Read the model definition and answer for the solid it produces. Units are mm, in the model's axes. A direction names the side the tool comes from. Coordinates: 2 decimals unless noted, no trailing zeros. Write each loop counter-clockwise with the first axis right and the second up, starting at its lowest first coordinate (ties: lowest second). Pieces come first, ordered by that corner, then holes.
(1) Section D-D on z = 4.75 is taken. State how many separate pieces and enclosed holes the cut face has, then the cut area to 3 significant figures.
(2) Given pin 1 (1 mm diameter, centred on y = -11, z = 1, fed in from +X); pin 2 (1.5 mm diameter, centred on x = 27, z = 0.5, fed in from -Y); pin 3 (1.8 mm diameter, centred on x = 4.5, z = 4, fed in from +Y), each flat-ended and moving along its own axis, determine where each tip first touches the part or whether it passes through.
(3) Find the intervals of material crossed by probe 1 along X at (y, z) = (-18, 4.25); probe 2 along X at (y, z) = (-8, 2.75); probe 3 along Y at (x, z) = (9, 1), in increasing order.
(4) Section A-A on y = 3 is taken. Write down the section's boundary in (x, z).
(5) The mould has two halves that part along X. Classify faces 4 (the flat face through (63.013, 1.422, 2.958)), 5 (the flat face through (3, -11, 0)), 6 (the cylindrical face through (-29.21, -4.43, 3.04)): +X half, -X half, draft (parallel to the pull), parting line (faces both ways), or undercut.
(6) Section C-C on x = 23 is taken. Write down the section's boundary in (y, z).
(7) Section B-B on x = -35.5 is taken. Write down the section's boundary in (y, z).
(8) Which of the six approach directions +Z, -Z, +X, -X, +Y, -Y give full straight-line access (tool end or side, diameter ignored) to faces 1 (the flat face through (56.063, -8.065, 3.042)), 2 (the cylindrical face through (-36.754, 13.724, 2.958)), 3 (the flat face through (-47.563, -31.236, 2.958))?
from build123d import *

# Parameters (mm, degrees)
SKETCH1_R                = 4.05
BOSS_EXTRUDE1_DEPTH      = 6
M4_CLEARANCE_HOLE1_D     = 4.5
M4_CLEARANCE_HOLE1_DEPTH = 80.96
M4_CLEARANCE_HOLE1_TIP   = 1.351936393
CUT_EXTRUDE1_DEPTH       = 103.314309644


with BuildPart() as part:
    # Sketch1 → Boss-Extrude1 (new body)
    with BuildSketch(Plane.XY):
        with BuildLine():
            Line((-65.19060966, -38.213571923), (-29.435009511, -24.059676563))
            ThreePointArc((-29.435009511, -24.059676563), (-26.147647316, -23.075006142), (-22.740346385, -22.666807174))
            Line((-22.740346385, -22.666807174), (18.034765948, -21.307032913))
            ThreePointArc((18.034765948, -21.307032913), (21.515927007, -21.494956503), (24.911568818, -22.284522385))
            Line((24.911568818, -22.284522385), (74.630790843, -38.525664943))
            ThreePointArc((74.630790843, -38.525664943), (93.086798158, -30.149764409), (86.35131748, -11.033979941))
            Line((86.35131748, -11.033979941), (39.011755224, 14.232375332))
            ThreePointArc((39.011755224, 14.232375332), (34.124223209, 16.06850435), (28.928004649, 16.57708242))
            Line((28.928004649, 16.57708242), (-31.672918815, 14.556154182))
            ThreePointArc((-31.672918815, 14.556154182), (-36.823710211, 13.702522548), (-41.578056522, 11.544854797))
            Line((-41.578056522, 11.544854797), (-78.64034873, -11.533366082))
            ThreePointArc((-78.64034873, -11.533366082), (-84.105870489, -31.018758249), (-65.19060966, -38.213571923))
        make_face()
        with Locations((-70.711551227, -24.266557754)):
            Circle(SKETCH1_R, mode=Mode.SUBTRACT)
        with Locations((79.288448772, -24.267115836)):
            Circle(SKETCH1_R, mode=Mode.SUBTRACT)
    extrude(amount=BOSS_EXTRUDE1_DEPTH)

    # M4 Clearance Hole1
    with Locations(Plane(origin=(-35.078495103, 7.961945554, 6), x_dir=(1, 0, 0), z_dir=(0, 0, 1))):
        with Locations((0, 0), (7.708679818, -25.162744902), (67.843830433, 2.262465733), (57.438792738, -23.51661265)):
            Hole(M4_CLEARANCE_HOLE1_D / 2, depth=M4_CLEARANCE_HOLE1_DEPTH)
            with Locations((0, 0, -(M4_CLEARANCE_HOLE1_DEPTH + M4_CLEARANCE_HOLE1_TIP / 2))):  # 118° drill point
                Cone(0, M4_CLEARANCE_HOLE1_D / 2, M4_CLEARANCE_HOLE1_TIP, mode=Mode.SUBTRACT)

    # Sketch4 → Cut-Extrude1 (cut, through all)
    with BuildSketch(Plane.XY.offset(6)):
        with BuildLine():
            Line((-59.730356843, -12.416942996), (-37.142655282, -1.702665692))
            ThreePointArc((-37.142655282, -1.702665692), (-29.150180354, -4.552287513), (-31.999802176, -12.544762441))
            Line((-31.999802176, -12.544762441), (-54.587503737, -23.259039746))
            ThreePointArc((-54.587503737, -23.259039746), (-62.579978665, -20.409417924), (-59.730356843, -12.416942996))
        make_face()
        with BuildLine():
            Line((63.134796659, -24.023141646), (40.065741433, -14.388895905))
            ThreePointArc((40.065741433, -14.388895905), (36.841387157, -6.540103673), (44.690179389, -3.315749397))
            Line((44.690179389, -3.315749397), (67.759234614, -12.949995138))
            ThreePointArc((67.759234614, -12.949995138), (70.983588891, -20.79878737), (63.134796659, -24.023141646))
        make_face()
        with BuildLine():
            Line((-12.5, 6), (12.5, 6))
            ThreePointArc((12.5, 6), (18.5, 0), (12.5, -6))
            Line((12.5, -6), (-12.5, -6))
            ThreePointArc((-12.5, -6), (-18.5, 0), (-12.5, 6))
        make_face()
    extrude(amount=-CUT_EXTRUDE1_DEPTH, mode=Mode.SUBTRACT)


solid = part.part
Response:
1. separate pieces: 1
1. enclosed holes: 9
1. area: 4,980 mm2
2. pin 1: stops at x = 87.16
2. pin 2: stops at y = -23.21
2. pin 3: stops at y = 15.79
3. probe 1: x = -84.34 to -63.16, -43.5 to -29.47, -25.27 to 48.71, 71.43 to 92.92
3. probe 2: x = -72.97 to -50.42, -28.64 to 36.44, 55.91 to 80.67
3. probe 3: y = -21.61 to -6, 6 to 15.91
4. outline: (-55.3, 0) - (-17.7, 0) - (-17.7, 6) - (-55.3, 6) - close; (17.7, 0) - (60.06, 0) - (60.06, 6) - (17.7, 6) - close
5. face 4: +X half
5. face 5: draft
5. face 6: undercut
6. outline: (-21.76, 0) - (-17.71, 0) - (-17.71, 6) - (-21.76, 6) - close; (-13.4, 0) - (16.38, 0) - (16.38, 6) - (-13.4, 6) - close
7. outline: (-26.46, 0) - (-14.21, 0) - (-14.21, 6) - (-26.46, 6) - close; (-1.2, 0) - (5.75, 0) - (5.75, 6) - (-1.2, 6) - close; (10.17, 0) - (14.06, 0) - (14.06, 6) - (10.17, 6) - close
8. face 1: +Z, -Z
8. face 2: +Z, -Z, -X, +Y
8. face 3: +Z, -Z, -Y
